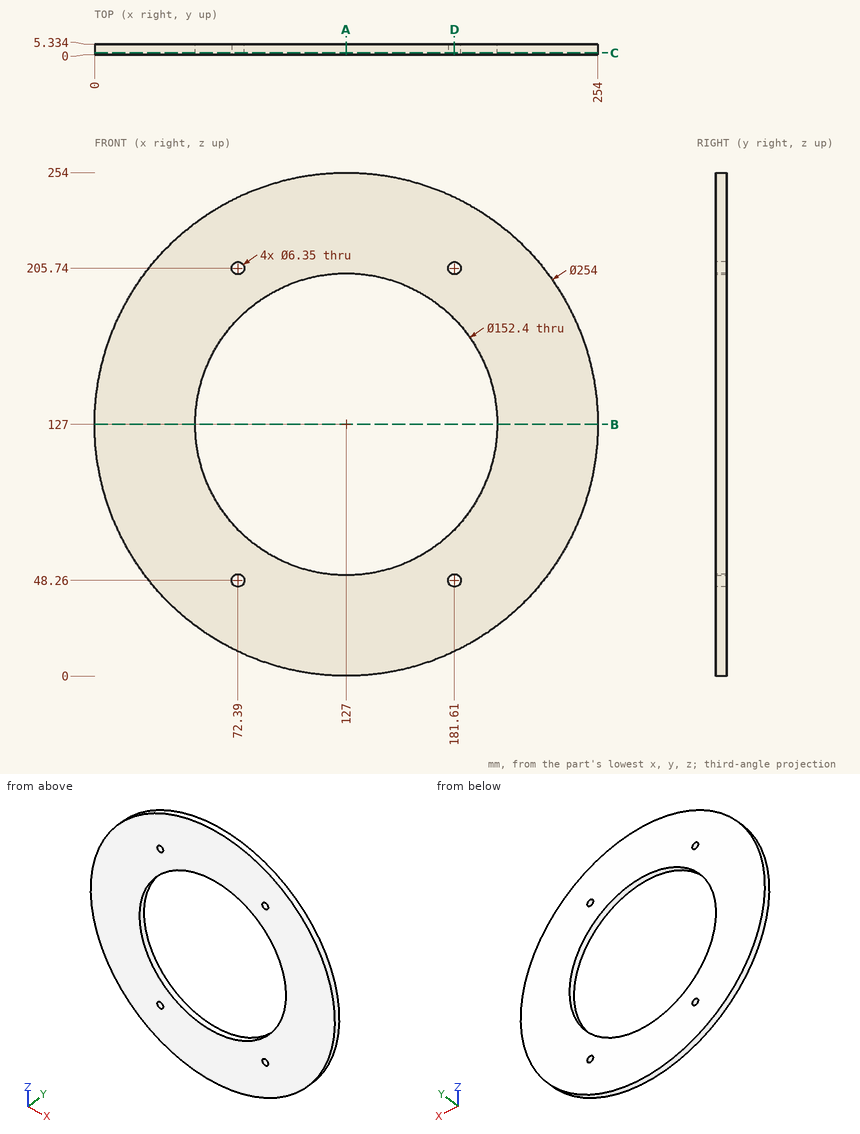
Part print with two shaded views. Sizes in mm from the minimum x, y, z corner. Coordinates: 2 decimals unless noted, no trailing zeros. Order: outer loops, then holes, each group sorted by start corner. A loop starts at its lowest first (then second) coordinate and runs counter-clockwise, first axis right, second up. Notation, with made-up numbers: M 83,14 L 100,14 A27 ccw 100,42 Z; hole C -19.75,-9 d5. An arc over 180 degrees is marked long. One line per question, with ' | ' between items. Start each with the question number.
1. Wall check: line 1 along X through (y, z) = (2.2, 127); line 2 along Z through (x, y) = (124.5, 2.95); line 3 along Z through (x, y) = (72.5, 2.45). Give the ranges that are in metal, low to high. Write a range as [from, to].
2. Cut at D-D (x = 181.61). Write the cut outline in (y, z) (3 decimals).
3. Flat gauge pins, fed straight in: P1, Ø5.5, axis at x = 72.39, z = 48.26, coming from the -Y side; P2, Ø2, axis at y = 0.5, z = 161, coming from the -X side; P3, Ø1, axis at x = 119.5, y = 5, coming from the +Z side; P4, Ø1, axis at y = 3.5, z = 220, coming from the +X side. Where does each tip first touch, or does it go through?
4. Cut at C-C (y = 0.85). Write the cut outline in (x, z) (3 decimals).
5. Cut at B-B (z = 127). Write the cut outline in (x, y), plus the area to 3 significant figures.
6. Cut at A-A (x = 127). Write the cut outline in (y, z), plus the area to 3 significant figures.
The answers:
1) line 1: x = [0, 50.8], [203.2, 254] | line 2: z = [0.02, 50.84], [203.16, 253.98] | line 3: z = [12.29, 45.09], [51.43, 73.74], [180.26, 202.57], [208.91, 241.71]
2) outline: M 0,12.341 L 5.334,12.341 L 5.334,45.085 L 0,45.085 Z; M 0,51.435 L 5.334,51.435 L 5.334,73.857 L 0,73.857 Z; M 0,180.143 L 5.334,180.143 L 5.334,202.565 L 0,202.565 Z; M 0,208.915 L 5.334,208.915 L 5.334,241.659 L 0,241.659 Z
3) P1: passes through | P2: stops at x = 4.36 | P3: stops at z = 253.81 | P4: stops at x = 214.02
4) outline: C 127,127 d254; hole C 127,127 d152.4; hole C 72.39,48.26 d6.35; hole C 72.39,205.74 d6.35; hole C 181.61,48.26 d6.35; hole C 181.61,205.74 d6.35
5) outline: M 0,0 L 50.8,0 L 50.8,5.33 L 0,5.33 Z; M 203.2,0 L 254,0 L 254,5.33 L 203.2,5.33 Z | area: 542 mm2
6) outline: M 0,0 L 5.33,0 L 5.33,50.8 L 0,50.8 Z; M 0,203.2 L 5.33,203.2 L 5.33,254 L 0,254 Z | area: 542 mm2
